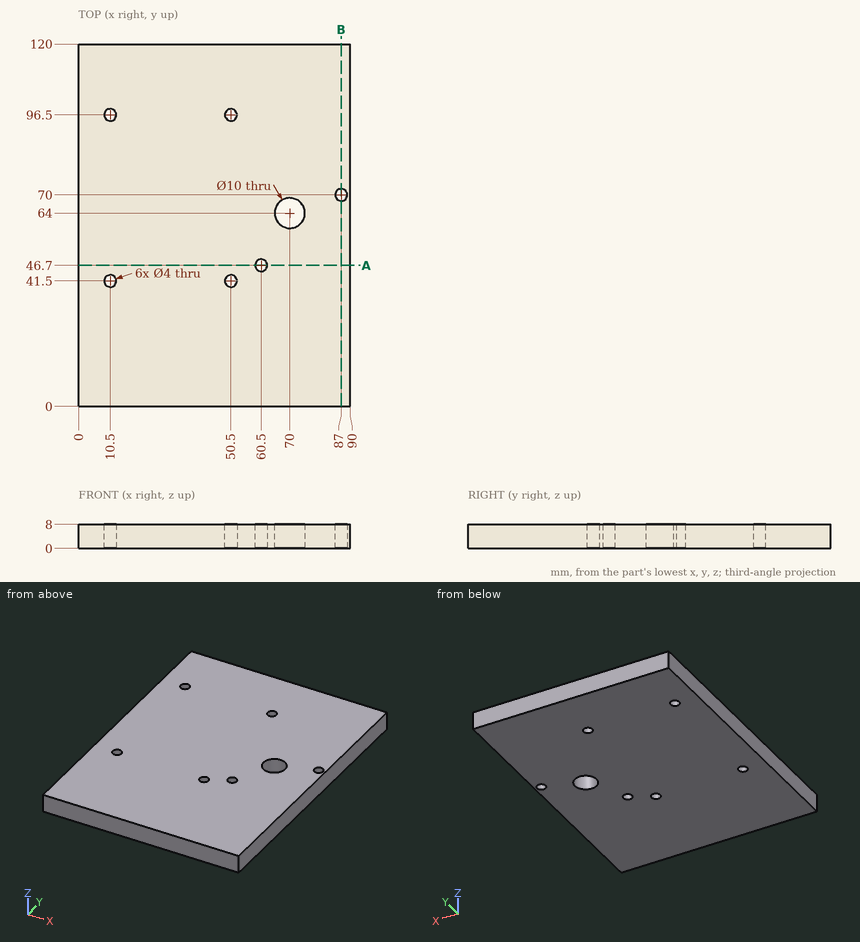
Drawing for the job (mm, zero at the part's lowest x, y, z). Give positions to 0.01 mm unless a question says otherwise; leave off trailing zeros. Loops run counter-clockwise (first coordinate to the right, second up) from the corner with the lowest first, then second, coordinate; pieces in that order, holes last. Notation, with made-up numbers: (35.5, -9) - (58.5, -9) arc R7 ccw to (58.5, 0) - close; hole circle Ø8 at (61.5, 40.5). An arc over 180 degrees is marked (long way). Write item = value, one per line. Start each with the question number.
1) Drop a flat-ended pin along its axis: pin 1 Ø2.5 at (x, y) = (50.5, 41.5) entering from +Z. Give the stop position or say it passes through.
2) Band-saw the part on A-A on y = 46.7. Give the cut face in (x, z).
3) Band-saw the part on B-B on x = 87. Give the cut face in (y, z).
4) Probe probe 1 along Y at (x, z) = (50.5, 4); probe 2 along X at (y, z) = (96, 6.5); probe 3 along Y at (x, z) = (70, 5.75). List the from-to ranges inside material, lowest first. Write a range as from..to.
Final values:
q1.pin_1 = through
q2.outline = (0, 0) - (58.5, 0) - (58.5, 8) - (0, 8) - close; (62.5, 0) - (90, 0) - (90, 8) - (62.5, 8) - close
q3.outline = (0, 0) - (68, 0) - (68, 8) - (0, 8) - close; (72, 0) - (120, 0) - (120, 8) - (72, 8) - close
q4.probe_1 = 0..39.5, 43.5..94.5, 98.5..120
q4.probe_2 = 0..8.56, 12.44..48.56, 52.44..90
q4.probe_3 = 0..59, 69..120
